from build123d import *

# Parameters (mm, degrees)
MODEL_R             = 1.499994887
BOSS_EXTRUDE1_DEPTH = 3


with BuildPart() as part:
    # Model → Boss-Extrude1 (new body)
    with BuildSketch(Plane.XY):
        with BuildLine():
            ThreePointArc((127.267167807, 75.815864008), (124.338313147, 82.886904548), (117.267301896, 85.815829919))
            Line((117.267301896, 85.815829919), (33.567587225, 85.815829919))
            ThreePointArc((33.567587225, 85.815829919), (26.851651545, 83.222459398), (23.567621314, 76.815860599))
            Line((23.567621314, 76.815860599), (23.567621314, 67.211322932))
            Line((23.567621314, 67.211322932), (23.567621314, 11.790716994))
            Line((23.567621314, 11.790716994), (23.567621314, 0.81611968))
            ThreePointArc((23.567621314, 0.81611968), (26.49658283, -6.254927716), (33.567648038, -9.183846231))
            Line((33.567648038, -9.183846231), (117.267301896, -9.183846231))
            ThreePointArc((117.267301896, -9.183846231), (124.338288146, -6.25489586), (127.267167807, 0.816119679))
            Line((127.267167807, 0.816119679), (127.267167807, 11.594182037))
            Line((127.267167807, 11.594182037), (127.267167807, 49.315954345))
            Line((127.267167807, 49.315954345), (127.267167807, 75.815864008))
        make_face()
        with Locations((33.567587225, 0.816119679)):
            Circle(MODEL_R, mode=Mode.SUBTRACT)
        with Locations((63.267605432, 16.315947389)):
            Circle(MODEL_R, mode=Mode.SUBTRACT)
        with Locations((117.267226438, 0.816095138)):
            Circle(MODEL_R, mode=Mode.SUBTRACT)
        with Locations((107.26755543, 16.315947389)):
            Circle(MODEL_R, mode=Mode.SUBTRACT)
        with Locations((63.267555431, 60.315947389)):
            Circle(MODEL_R, mode=Mode.SUBTRACT)
        with Locations((33.610039072, 75.815864008)):
            Circle(MODEL_R, mode=Mode.SUBTRACT)
        with BuildLine():
            Line((53.483284952, 45.387404724), (75.735868353, 67.640059648))
            Line((75.735868353, 67.640059648), (82.064163104, 73.968374739))
            Line((82.064163104, 73.968374739), (85.267424216, 77.171646146))
            Line((85.267424216, 77.171646146), (89.463558538, 72.975511824))
            Line((89.463558538, 72.975511824), (122.001384869, 40.437685493))
            ThreePointArc((122.001384869, 40.437685493), (122.88006153, 38.316372381), (122.001384869, 36.195059268))
            Line((122.001384869, 36.195059268), (87.388740737, 1.582415136))
            ThreePointArc((87.388740737, 1.582415136), (85.267425214, 0.703738475), (83.146111103, 1.582418545))
            Line((83.146111103, 1.582418545), (53.483284952, 31.245340037))
            ThreePointArc((53.483284952, 31.245340037), (50.554374112, 38.316372381), (53.483284952, 45.387404724))
        make_face(mode=Mode.SUBTRACT)
        with Locations((107.26755543, 60.315797391)):
            Circle(MODEL_R, mode=Mode.SUBTRACT)
        with Locations((117.267226438, 75.815864008)):
            Circle(MODEL_R, mode=Mode.SUBTRACT)
    extrude(amount=BOSS_EXTRUDE1_DEPTH)


solid = part.part
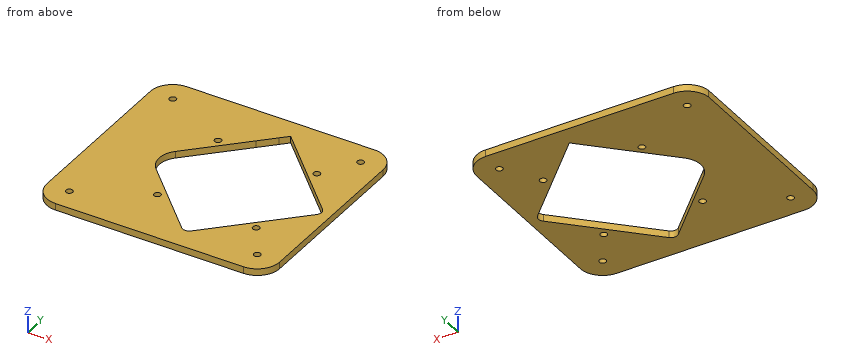
Verification items for the finished model (mm, model axes). Coordinates: 2 decimals unless noted, no trailing zeros. Loops run counter-clockwise (first coordinate to the right, second up) from the corner with the lowest first, then second, coordinate; pieces in that order, holes last. Notation, with made-up numbers: (79, 14.25) -> (84, 14.25) arc R24 cw to (84, 25.25) -> close; hole circle Ø4 at (-11, 28.25). An arc over 180 degrees is marked (long way). Answer as a JSON object with one key per item and string values. Group by question number.
Item 1: Depth check by flat-ended pin: pin 1 (5 mm diameter, centred on x = 117.27, y = 0.82, fed in from -Z). Enter the tip coordinate at first touch or a pass-through.
Item 2: Sectioned sample at A-A on y = 44. Record the boundary of the cut face in (x, z), plus the area to 3 significant figures.
Item 3: Sectioned sample at C-C on y = 24. Record the boundary of the cut face in (x, z).
Item 4: Scan lines: probe 1 along X at (y, z) = (76.5, 2.8); probe 2 along Y at (x, z) = (34.5, 2.35); probe 3 along X at (y, z) = (74.5, 0.8). Record each from-to range of solid material in increasing order.
Item 5: Sectioned sample at B-B on z = 1.05. State how many separate pieces and enclosed holes the cut face has, plus the area to 3 significant figures.
Evaluation:
{
 "1": {"pin 1": "stops at z = 0"},
 "2": {"outline": "(23.57, 0) -> (52.33, 0) -> (52.33, 3) -> (23.57, 3) -> close; (118.44, 0) -> (127.27, 0) -> (127.27, 3) -> (118.44, 3) -> close", "area": "113 mm²"},
 "3": {"outline": "(23.57, 0) -> (60.73, 0) -> (60.73, 3) -> (23.57, 3) -> close; (109.81, 0) -> (127.27, 0) -> (127.27, 3) -> (109.81, 3) -> close"},
 "4": {"probe 1": "x = 23.57 to 32.28, 34.94 to 84.6, 85.94 to 115.93, 118.6 to 127.24", "probe 2": "y = -9.18 to -0.36, 1.99 to 74.61, 77.02 to 85.82", "probe 3": "x = 23.57 to 32.89, 34.33 to 82.6, 87.94 to 116.55, 117.99 to 127.27"},
 "5": {"separate pieces": "1", "enclosed holes": "9", "area": "6,720 mm²"}
}
